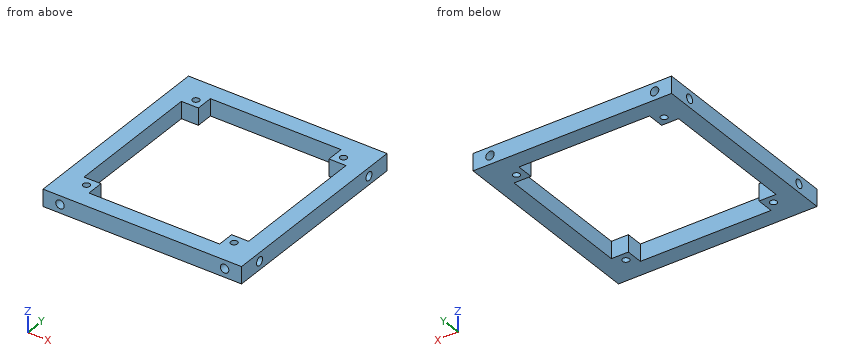
from build123d import *

# Parameters (mm, degrees)
SKETCH1_W          = 46.8
SKETCH1_H          = 48.4
SKETCH1_R          = 0.8
LEFT_PANEL_DEPTH   = 4
SKETCH9_R          = 1
CUT_EXTRUDE5_DEPTH = 4
SKETCH10_R         = 1
CUT_EXTRUDE6_DEPTH = 4
SKETCH11_R         = 1
CUT_EXTRUDE7_DEPTH = 4
SKETCH12_R         = 1
CUT_EXTRUDE8_DEPTH = 4


with BuildPart() as part:
    # Sketch1 → left_panel (new body)
    with BuildSketch(Plane.XY):
        with Locations((23.4, 24.2)):
            Rectangle(SKETCH1_W, SKETCH1_H)
        with Locations((6, 6)):
            Circle(SKETCH1_R, mode=Mode.SUBTRACT)
        with Locations((40.8, 6)):
            Circle(SKETCH1_R, mode=Mode.SUBTRACT)
        with Locations((40.8, 42.4)):
            Circle(SKETCH1_R, mode=Mode.SUBTRACT)
        with Locations((6, 42.4)):
            Circle(SKETCH1_R, mode=Mode.SUBTRACT)
        Polygon((8, 44.4), (38.8, 44.4), (38.8, 40.4), (42.8, 40.4), (42.8, 8), (38.8, 8), (38.8, 4), (8, 4), (8, 8), (4, 8), (4, 40.4), (8, 40.4), align=None, mode=Mode.SUBTRACT)
    extrude(amount=LEFT_PANEL_DEPTH)

    # Sketch9 → Cut-Extrude5 (cut)
    with BuildSketch(Plane(origin=(46.8, 0, 0), x_dir=(0, 0, -1), z_dir=(1, 0, 0))):
        with Locations((-2, 6)):
            Circle(SKETCH9_R)
        with Locations((-2, 42.4)):
            Circle(SKETCH9_R)
    extrude(amount=-CUT_EXTRUDE5_DEPTH, mode=Mode.SUBTRACT)

    # Sketch10 → Cut-Extrude6 (cut)
    with BuildSketch(Plane.ZY):
        with Locations((2, 6)):
            Circle(SKETCH10_R)
        with Locations((2, 42.4)):
            Circle(SKETCH10_R)
    extrude(amount=-CUT_EXTRUDE6_DEPTH, mode=Mode.SUBTRACT)

    # Sketch11 → Cut-Extrude7 (cut)
    with BuildSketch(Plane(origin=(0, 48.4, 0), x_dir=(1, 0, 0), z_dir=(0, 1, 0))):
        with Locations((4, -2)):
            Circle(SKETCH11_R)
        with Locations((42.8, -2)):
            Circle(SKETCH11_R)
    extrude(amount=-CUT_EXTRUDE7_DEPTH, mode=Mode.SUBTRACT)

    # Sketch12 → Cut-Extrude8 (cut)
    with BuildSketch(Plane.XZ):
        with Locations((4, 2)):
            Circle(SKETCH12_R)
        with Locations((42.8, 2)):
            Circle(SKETCH12_R)
    extrude(amount=-CUT_EXTRUDE8_DEPTH, mode=Mode.SUBTRACT)


solid = part.part
Verification items for the finished model (mm, model axes). Give positions to 0.01 mm unless a question says otherwise; leave off trailing zeros. Order: outer loops, then holes, each group sorted by start corner. A loop starts at its lowest first (then second) coordinate and runs counter-clockwise, first axis right, second up. Notation, with made-up numbers: M 49.25,39 L 54.25,39 A32 cw 54.25,70 Z; hole C -5,3 d4. An arc over 180 degrees is marked long. Answer as a JSON object with one key per item and string values. Group by question number.
1) Scan lines: line 1 along X through (y, z) = (42.5, 0.45); line 2 along X through (y, z) = (42.4, 2.75); line 3 along Y through (x, z) = (40.8, 2.15). Record each from-to range of solid material in increasing order. Write a range as [from, to].
2) Cross-section at B-B (x = 38). Enter the section's corners in (y, z).
3) Cross-section at C-C (y = 14.5). Enter the section's corners in (x, z).
4) Depth check by flat-ended pin: pin 1 Ø1.6 at (x, z) = (4, 2) entering from -Y; pin 2 Ø3 at (x, y) = (28.5, 6.5) entering from -Z. Enter the tip coordinate at first touch or a pass-through.
5) Cross-section at A-A (y = 42.4). Enter the section's corners in (x, z), then the cut area to 3 significant figures.
6) Cross-section at D-D (x = 6). Enter the section's corners in (y, z).
Result sheet:
{
 "1": {"line 1": "x = [0, 5.21], [6.79, 8], [38.8, 40.01], [41.59, 46.8]", "line 2": "x = [4, 5.2], [6.8, 8], [38.8, 40], [41.6, 42.8]", "line 3": "y = [0, 5.2], [6.8, 8], [40.4, 41.6], [43.2, 48.4]"},
 "2": {"outline": "M 0,0 L 4,0 L 4,4 L 0,4 Z; M 44.4,0 L 48.4,0 L 48.4,4 L 44.4,4 Z"},
 "3": {"outline": "M 0,0 L 4,0 L 4,4 L 0,4 Z; M 42.8,0 L 46.8,0 L 46.8,4 L 42.8,4 Z"},
 "4": {"pin 1": "stops at y = 4", "pin 2": "passes through"},
 "5": {"outline": "M 0,0 L 5.2,0 L 5.2,4 L 0,4 L 0,3 L 4,3 L 4,1 L 0,1 Z; M 6.8,0 L 8,0 L 8,4 L 6.8,4 Z; M 38.8,0 L 40,0 L 40,4 L 38.8,4 Z; M 41.6,0 L 46.8,0 L 46.8,1 L 42.8,1 L 42.8,3 L 46.8,3 L 46.8,4 L 41.6,4 Z", "area": "35.2 mm2"},
 "6": {"outline": "M 0,0 L 5.2,0 L 5.2,4 L 0,4 Z; M 6.8,0 L 8,0 L 8,4 L 6.8,4 Z; M 40.4,0 L 41.6,0 L 41.6,4 L 40.4,4 Z; M 43.2,0 L 48.4,0 L 48.4,4 L 43.2,4 Z"}
}
